from build123d import *

# Parameters (mm, degrees)
SKETCH1_W           = 260
SKETCH1_H           = 260
SKETCH1_R           = 1.55
SKETCH1_R_2         = 1.5875
SKETCH1_R_3         = 1.6
SKETCH1_R_4         = 1.7
SKETCH1_R_5         = 3.175
SKETCH1_R_6         = 2.415
SKETCH1_R_7         = 1.651
BOSS_EXTRUDE2_DEPTH = 6.35
SKETCH2_R           = 1.5875
CUT_EXTRUDE1_DEPTH  = 7.35
SKETCH3_R           = 3.175
CUT_EXTRUDE2_DEPTH  = 7.35


with BuildPart() as part:
    # Sketch1 → Boss-Extrude2 (new body)
    with BuildSketch(Plane.XY):
        Rectangle(SKETCH1_W, SKETCH1_H)
        with Locations((-26.035, 26.67)):
            Circle(SKETCH1_R, mode=Mode.SUBTRACT)
        with Locations((-26.035, -26.67)):
            Circle(SKETCH1_R, mode=Mode.SUBTRACT)
        with Locations((26.035, 26.67)):
            Circle(SKETCH1_R, mode=Mode.SUBTRACT)
        with Locations((26.035, -26.67)):
            Circle(SKETCH1_R, mode=Mode.SUBTRACT)
        with Locations((-116.825, 25.402702903)):
            Circle(SKETCH1_R_2, mode=Mode.SUBTRACT)
        with Locations((-113.65, -40.635194695)):
            Circle(SKETCH1_R_2, mode=Mode.SUBTRACT)
        with Locations((-68.565, 25.404805305)):
            Circle(SKETCH1_R_2, mode=Mode.SUBTRACT)
        with Locations((-37, 117)):
            Circle(SKETCH1_R_3, mode=Mode.SUBTRACT)
        with Locations((-37, 83)):
            Circle(SKETCH1_R_3, mode=Mode.SUBTRACT)
        with Locations((-3.5, 117)):
            Circle(SKETCH1_R_3, mode=Mode.SUBTRACT)
        with Locations((-3.5, 83)):
            Circle(SKETCH1_R_3, mode=Mode.SUBTRACT)
        with Locations((3.5, 117)):
            Circle(SKETCH1_R_3, mode=Mode.SUBTRACT)
        with Locations((37, 117)):
            Circle(SKETCH1_R_3, mode=Mode.SUBTRACT)
        with Locations((37, 83)):
            Circle(SKETCH1_R_3, mode=Mode.SUBTRACT)
        with Locations((3.5, 83)):
            Circle(SKETCH1_R_3, mode=Mode.SUBTRACT)
        with Locations((-13.25, -65.25)):
            Circle(SKETCH1_R_4, mode=Mode.SUBTRACT)
        with Locations((13.25, -65.25)):
            Circle(SKETCH1_R_4, mode=Mode.SUBTRACT)
        with Locations((13.25, -94.75)):
            Circle(SKETCH1_R_4, mode=Mode.SUBTRACT)
        with Locations((-13.25, -94.75)):
            Circle(SKETCH1_R_4, mode=Mode.SUBTRACT)
        with Locations((-76.33, 76.33)):
            Circle(SKETCH1_R_5, mode=Mode.SUBTRACT)
        with Locations((0, 55.575)):
            Circle(SKETCH1_R_6, mode=Mode.SUBTRACT)
        with Locations((-55.575, 0)):
            Circle(SKETCH1_R_6, mode=Mode.SUBTRACT)
        with Locations((0, -55.575)):
            Circle(SKETCH1_R_6, mode=Mode.SUBTRACT)
        with Locations((55.575, 0)):
            Circle(SKETCH1_R_6, mode=Mode.SUBTRACT)
        with Locations((-39.297459364, 39.297459364)):
            Circle(SKETCH1_R_6, mode=Mode.SUBTRACT)
        with Locations((39.297459364, 39.297459364)):
            Circle(SKETCH1_R_6, mode=Mode.SUBTRACT)
        with Locations((39.297459364, -39.297459364)):
            Circle(SKETCH1_R_6, mode=Mode.SUBTRACT)
        with Locations((-39.297459364, -39.297459364)):
            Circle(SKETCH1_R_6, mode=Mode.SUBTRACT)
        with Locations((76.33, 76.33)):
            Circle(SKETCH1_R_5, mode=Mode.SUBTRACT)
        with Locations((76.33, -76.33)):
            Circle(SKETCH1_R_5, mode=Mode.SUBTRACT)
        with Locations((-76.33, -76.33)):
            Circle(SKETCH1_R_5, mode=Mode.SUBTRACT)
        with Locations((-71.74, -40.635194695)):
            Circle(SKETCH1_R_2, mode=Mode.SUBTRACT)
        with Locations((6.35, -121.3)):
            Circle(SKETCH1_R_7, mode=Mode.SUBTRACT)
        with Locations((-6.35, -121.3)):
            Circle(SKETCH1_R_7, mode=Mode.SUBTRACT)
        with Locations((121.3, 126.35)):
            Circle(SKETCH1_R_7, mode=Mode.SUBTRACT)
        with Locations((121.3, 113.65)):
            Circle(SKETCH1_R_7, mode=Mode.SUBTRACT)
    extrude(amount=BOSS_EXTRUDE2_DEPTH)

    # Sketch2 → Cut-Extrude1 (cut, through all)
    with BuildSketch(Plane(origin=(0, 0, 0), x_dir=(-1, 0, 0), z_dir=(0, 0, -1))):
        with Locations((0, 19.05)):
            Circle(SKETCH2_R)
        with Locations((-19.05, 0)):
            Circle(SKETCH2_R)
        with Locations((19.05, 0)):
            Circle(SKETCH2_R)
        with Locations((0, -19.05)):
            Circle(SKETCH2_R)
    extrude(amount=-CUT_EXTRUDE1_DEPTH, mode=Mode.SUBTRACT)

    # Sketch3 → Cut-Extrude2 (cut, through all)
    with BuildSketch(Plane(origin=(0, 0, 0), x_dir=(-1, 0, 0), z_dir=(0, 0, -1))):
        with Locations((-19.05, 19.05)):
            Circle(SKETCH3_R)
        with Locations((19.05, 19.05)):
            Circle(SKETCH3_R)
        with Locations((-19.05, -19.05)):
            Circle(SKETCH3_R)
        with Locations((19.05, -19.05)):
            Circle(SKETCH3_R)
    extrude(amount=-CUT_EXTRUDE2_DEPTH, mode=Mode.SUBTRACT)


solid = part.part
Design review of the part built by this model. Coordinates are the model's own, in mm. Give positions to 0.01 mm unless a question says otherwise; leave off trailing zeros. Loops run counter-clockwise (first coordinate to the right, second up) from the corner with the lowest first, then second, coordinate; pieces in that order, holes last. Notation, with made-up numbers: M -19.5,27.25 L -13.5,27.25 A15 cw -13.5,53.25 Z; hole C 55.25,35 d6. An arc over 180 degrees is marked long. One line per question, with ' | ' between items. Start each with the question number.
1. To check wall thickness, follow L1, parallel to Y at x = 121.3, z = 2; L2, parallel to Y at x = 26.5, z = 4.75; L3, parallel to X at y = 117, z = 4.5. State the ranges of each line that lie inside material, in increasing order.
2. Add section A-A (x = -76.33). Write out the cut boundary in (y, z) (3 decimals), plus the area to 3 significant figures.
3. The part is to be moulded in two halves that separate along X. For faces 1 (the face through (78.037, 79.007, 3.131)), 2 (the face through (-2, -130, 3)), 3 (the face through (-130, -2, 3)), say which applies: released by +X, released by -X, zero draft, split by the parting line, or undercut.
4. Insertion check: P1, Ø10, axis at x = -76.33, y = 76.33, coming from the -Z side. The pin has a flat end and moves straight along its axis. Give the tip position at first contact, or say it passes through.
Worked out:
1) L1: y = -130 to 112, 115.3 to 124.7, 128 to 130 | L2: y = -130 to -28.15, -25.19 to 25.19, 28.15 to 130 | L3: x = -130 to -38.6, -35.4 to -5.1, -1.9 to 1.9, 5.1 to 35.4, 38.6 to 130
2) outline: M -130,0 L -79.505,0 L -79.505,6.35 L -130,6.35 Z; M -73.155,0 L 73.155,0 L 73.155,6.35 L -73.155,6.35 Z; M 79.505,0 L 130,0 L 130,6.35 L 79.505,6.35 Z | area: 1,570 mm²
3) face 1: undercut | face 2: zero draft | face 3: released by -X
4) P1: stops at z = 0
